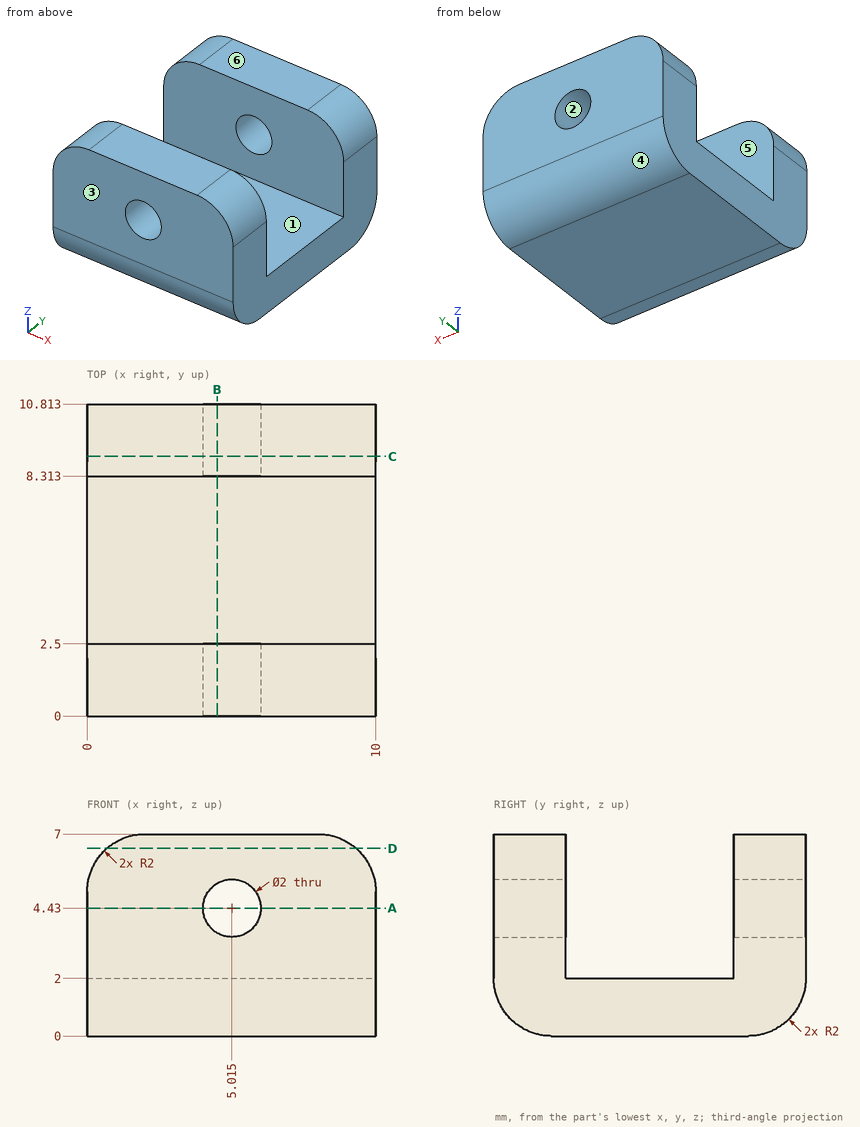
Source: three-view drawing plus pictorial views. Frame: mm from the lowest corner of the part. A direction names the side the tool comes from. Coordinates: 2 decimals unless noted, no trailing zeros. Write each loop counter-clockwise with the first axis right and the second up, starting at its lowest first coordinate (ties: lowest second). Pieces come first, ordered by that corner, then holes. Notation, with made-up numbers: (19, 35.25) - (48, 35.25) arc R13 cw to (48, 53.25) - close; hole circle Ø8 at (67, 8). An arc over 180 degrees is marked (long way). Return JSON: item names as keys, results as strings.
Item 1: Section query D-D (z = 6.5). Output: boundary loops of the cut face in (x, y).
Completed:
{"outline": "(0.68, 0) - (9.32, 0) - (9.32, 2.5) - (0.68, 2.5) - close; (0.68, 8.31) - (9.32, 8.31) - (9.32, 10.81) - (0.68, 10.81) - close"}
Item 2: Section query A-A (z = 4.43). Output: boundary loops of the cut face in (x, y) (1 decimal).
Completed:
{"outline": "(0, 0) - (4, 0) - (4, 2.5) - (0, 2.5) - close; (0, 8.3) - (4, 8.3) - (4, 10.8) - (0, 10.8) - close; (6, 0) - (10, 0) - (10, 2.5) - (6, 2.5) - close; (6, 8.3) - (10, 8.3) - (10, 10.8) - (6, 10.8) - close"}
Item 3: Pull-direction query (Y, two-part tool) for the marked faces 3, 4, 5 and 6; classes: +Y half, -Y half, draft (parallel to the pull), parting line (faces both ways), or undercut.
Completed:
{"face 3": "-Y half", "face 4": "+Y half", "face 5": "undercut", "face 6": "draft"}
Item 4: Reachability of the marked faces 1 and 2 from +Z, -Z, +X, -X, +Y, -Y: full face, straight path, thin tool, end or side. Return the list, or none.
Completed:
{"face 1": "+Z, +X, -X", "face 2": "+Y, -Y"}
Item 5: Section query B-B (x = 4.5). Output: boundary loops of the cut face in (y, z).
Completed:
{"outline": "(0, 2) arc R2 ccw to (2, 0) - (8.81, 0) arc R2 ccw to (10.81, 2) - (10.81, 3.57) - (8.31, 3.57) - (8.31, 2) - (2.5, 2) - (2.5, 3.57) - (0, 3.57) - close; (0, 5.29) - (2.5, 5.29) - (2.5, 7) - (0, 7) - close; (8.31, 5.29) - (10.81, 5.29) - (10.81, 7) - (8.31, 7) - close"}
Item 6: Line query: L1, parallel to Y at x = 7.25, z = 5.75; L2, parallel to X at y = 10.15, z = 4.43 (1 decimal); L3, parallel to Z at x = 9, y = 7.5. Output: solid intervals per line, ascending.
Completed:
{"L1": "y = 0 to 2.5, 8.31 to 10.81", "L2": "x = 0 to 4, 6 to 10", "L3": "z = 0 to 2"}
Item 7: Section query C-C (y = 9). Output: boundary loops of the cut face in (x, z) (1 decimal).
Completed:
{"outline": "(0, 0) - (10, 0) - (10, 5) arc R2 ccw to (8, 7) - (2, 7) arc R2 ccw to (0, 5) - close; hole circle Ø2 at (5, 4.4)"}
Item 8: Pin query (flat end, axial travel): pin 1 Ø1.8 at (x, z) = (5.01, 4.43) entering from +Y; pin 2 Ø1 at (x, y) = (5, 6) entering from +Z. Return the tip coordinate at first contact, or that it passes through.
Completed:
{"pin 1": "passes through", "pin 2": "stops at z = 2"}
